Could you check a few things on this model? Use its own coordinates, in mm. A direction names the side the tool comes from. Round coordinates to 2 decimals unless told otherwise and drop trailing zeros. Loops run counter-clockwise (first coordinate to the right, second up) from the corner with the lowest first, then second, coordinate; pieces in that order, holes last. Notation, with made-up numbers: (-31.75, 56.25) - (18.25, 56.25) arc R6 cw to (18.25, 64.25) - close; hole circle Ø6 at (10.5, -8). An arc over 180 degrees is marked (long way). Use one line per item in the form item = value.
```python
from build123d import *

# Parameters (mm, degrees)
SKETCH_1_R      = 3.6
SKETCH_1_R_2    = 2.3
EXTRUDE_1_DEPTH = 5
EXTRUDE_START   = 5
SKETCH_1_8_R    = 3.6
EXTRUDE_2_DEPTH = 20
FILLET_2_R      = 10
FILLET_3_R      = 3


with BuildPart() as part:
    # 草图1 → 凸台-拉伸1 (new body)
    # profile 1 of 5: a face of its own
    with BuildSketch(Plane(origin=(0, 0, 5), x_dir=(1, 0, 0), z_dir=(0, 1, 0))):
        with BuildLine():
            ThreePointArc((13, -81.528896907), (0, -82.5), (-13, -81.528896907))
            Line((-13, -81.528896907), (-13, -94.528896907))
            Line((-13, -94.528896907), (13, -94.528896907))
            Line((13, -94.528896907), (13, -81.528896907))
        make_face()
        with Locations((-8, -89.528896907)):
            Circle(SKETCH_1_R, mode=Mode.SUBTRACT)
        with Locations((8, -89.528896907)):
            Circle(SKETCH_1_R, mode=Mode.SUBTRACT)
    # profile 2 of 5: a face of its own
    with BuildSketch(Plane(origin=(0, 0, 5), x_dir=(1, 0, 0), z_dir=(0, 1, 0))):
        with BuildLine():
            ThreePointArc((-83.157982179, 20), (0, -79.5), (83.157982179, 20))
            Line((83.157982179, 20), (86.204698248, 20))
            ThreePointArc((86.204698248, 20), (0, -82.5), (-86.204698248, 20))
            Line((-86.204698248, 20), (-83.157982179, 20))
        make_face()
    # profile 3 of 5: a face of its own
    with BuildSketch(Plane(origin=(0, 0, 5), x_dir=(1, 0, 0), z_dir=(0, 1, 0))):
        with BuildLine():
            ThreePointArc((13, -81.528896907), (0, -82.5), (-13, -81.528896907))
            Line((-13, -81.528896907), (-13, -94.528896907))
            Line((-13, -94.528896907), (13, -94.528896907))
            Line((13, -94.528896907), (13, -81.528896907))
        make_face()
        with Locations((-8, -89.528896907)):
            Circle(SKETCH_1_R, mode=Mode.SUBTRACT)
        with Locations((8, -89.528896907)):
            Circle(SKETCH_1_R, mode=Mode.SUBTRACT)
    # profile 4 of 5: a face of its own
    with BuildSketch(Plane(origin=(0, 0, 5), x_dir=(1, 0, 0), z_dir=(0, 1, 0))):
        with Locations((-8, -89.528896907)):
            Circle(SKETCH_1_R)
        with Locations(Location((-8, -89.528896907, 0), (0, 0, 270))):
            Circle(SKETCH_1_R_2, mode=Mode.SUBTRACT)
    # profile 5 of 5: a face of its own
    with BuildSketch(Plane(origin=(0, 0, 5), x_dir=(1, 0, 0), z_dir=(0, 1, 0))):
        with Locations((8, -89.528896907)):
            Circle(SKETCH_1_R)
        with Locations(Location((8, -89.528896907, 0), (0, 0, 270))):
            Circle(SKETCH_1_R_2, mode=Mode.SUBTRACT)
    extrude(amount=EXTRUDE_1_DEPTH)

    # 草图1<8> → 凸台-拉伸2 (add)
    # profile 1 of 3: a face of its own
    with BuildSketch(Plane(origin=(0, 0, 5), x_dir=(1, 0, 0), z_dir=(0, 1, 0)).offset(EXTRUDE_START)):
        with BuildLine():
            ThreePointArc((13, -81.528896907), (0, -82.5), (-13, -81.528896907))
            Line((-13, -81.528896907), (-13, -94.528896907))
            Line((-13, -94.528896907), (13, -94.528896907))
            Line((13, -94.528896907), (13, -81.528896907))
        make_face()
        with Locations(Location((-8, -89.528896907, 0), (0, 0, 270))):
            Circle(SKETCH_1_8_R, mode=Mode.SUBTRACT)
        with Locations(Location((8, -89.528896907, 0), (0, 0, 270))):
            Circle(SKETCH_1_8_R, mode=Mode.SUBTRACT)
    # profile 2 of 3: a face of its own
    with BuildSketch(Plane(origin=(0, 0, 5), x_dir=(1, 0, 0), z_dir=(0, 1, 0)).offset(EXTRUDE_START)):
        with BuildLine():
            ThreePointArc((-83.157982179, 20), (0, -79.5), (83.157982179, 20))
            Line((83.157982179, 20), (86.204698248, 20))
            ThreePointArc((86.204698248, 20), (0, -82.5), (-86.204698248, 20))
            Line((-86.204698248, 20), (-83.157982179, 20))
        make_face()
    # profile 3 of 3: a face of its own
    with BuildSketch(Plane(origin=(0, 0, 5), x_dir=(1, 0, 0), z_dir=(0, 1, 0)).offset(EXTRUDE_START)):
        with BuildLine():
            ThreePointArc((13, -81.528896907), (0, -82.5), (-13, -81.528896907))
            Line((-13, -81.528896907), (-13, -94.528896907))
            Line((-13, -94.528896907), (13, -94.528896907))
            Line((13, -94.528896907), (13, -81.528896907))
        make_face()
        with Locations(Location((-8, -89.528896907, 0), (0, 0, 270))):
            Circle(SKETCH_1_8_R, mode=Mode.SUBTRACT)
        with Locations(Location((8, -89.528896907, 0), (0, 0, 270))):
            Circle(SKETCH_1_8_R, mode=Mode.SUBTRACT)
    extrude(amount=EXTRUDE_2_DEPTH)

    # 圆角2
    # the kernel refuses this fillet: 10 mm, written as the material it adds along each edge
    with BuildSketch(Plane(origin=(13, 25, 86.528896907), x_dir=(0, 0, 1), z_dir=(0, -1, 0))) as fillet_2_piece_1:
        with BuildLine():
            CenterArc((8.219454002, -10), FILLET_2_R, 90, 76.355470557)
            ThreePointArc((-1.498325579, -7.641025641), (-0.664124715, -3.837187901), (0, 0))
            Line((0, 0), (8.219454002, 0))
        make_face()
    extrude(amount=25)
    with BuildSketch(Plane(origin=(-13, 25, 86.528896907), x_dir=(-0.9813116821933555, 0, -0.1924250045884026), z_dir=(0, -1, 0))) as fillet_2_piece_2:
        with BuildLine():
            CenterArc((8.231488348, -9.990096279), FILLET_2_R, 92.550190808, 76.355470557)
            Line((-1.581628474, -8.065846233), (0, 0))
            ThreePointArc((0, 0), (3.893271516, -0.086657558), (7.786543032, 0))
        make_face()
    extrude(amount=25)
    # the kernel refuses this fillet: 10 mm, written as the material it takes off along each edge
    with BuildSketch(Plane(origin=(-83.157982179, -17.895247065, -15), x_dir=(-0.13567256273252146, 0, 0.9907537311166635), z_dir=(0, 1, 0))) as fillet_2_2_piece_1:
        with BuildLine():
            CenterArc((7.581654969, -9.991025983), FILLET_2_R, 92.427524139, 43.365844963)
            Line((0.413355777, -3.018545313), (0, 0))
            ThreePointArc((0, 0), (3.579049413, -0.075830444), (7.158098826, 0))
        make_face()
    extrude(amount=60.790494129, mode=Mode.SUBTRACT)
    with BuildSketch(Plane(origin=(83.157982179, -17.895247065, -15), x_dir=(1, 0, 0), z_dir=(0, 1, 0))) as fillet_2_2_piece_2:
        with BuildLine():
            CenterArc((10.92726883, -6.15604485), FILLET_2_R, 142.004143618, 43.365844963)
            ThreePointArc((0.971157612, -7.091913119), (0.560708101, -3.535668449), (0, 0))
            Line((0, 0), (3.046716069, 0))
        make_face()
    extrude(amount=60.790494129, mode=Mode.SUBTRACT)

    # 圆角3
    fillet_3_edges = [part.edges().sort_by_distance(p)[0] for p in [
        (13, 12.5, 99.528896907),
        (-13, 12.5, 99.528896907),
    ]]
    fillet(fillet_3_edges, radius=FILLET_3_R)


solid = part.part
```
1. We'd pull the mould along Z, two halves only. Please class faces 3 (the face through (-7.842, 14.86, 90.932)), 4 (the face through (15.08, 12.68, 88.64)), 5 (the face through (-11, 25, 87)): +Z half, -Z half, draft (parallel to the pull), parting line (faces both ways), or undercut.
Solution:
face_3 = undercut
face_4 = +Z half
face_5 = draft
2. If we section it at D-D, the plane z = 35: Write out the boundary of the cut face in (x, y), plus the area to 3 significant figures.
Solution:
outline = (-80.2, 0) - (-76.91, 0) - (-76.91, 25) - (-80.2, 25) - close; (76.91, 0) - (80.2, 0) - (80.2, 25) - (76.91, 25) - close
area = 164 mm^2
3. For P1, Ø1.5, axis at y = 18, z = 40, coming from the -X side; P2, Ø2, axis at y = 19.5, z = 10.5, coming from the +X side; P3, Ø5, axis at y = 10, z = 62, coming from the +X side, each with a flat end and sliding along its axis, tell me the tip position at first contact or that it passes through.
Solution:
P1 = -78.2
P2 = 86.98
P3 = 64.16
4. If we section it at B-B, the plane x = 8: Write out the boundary of the cut face in (y, z), plus the area to 3 significant figures.
Solution:
outline = (0, 84.12) - (25, 84.12) - (25, 90.93) - (5, 90.93) - (5, 92.23) - (0, 92.23) - close; (0, 96.83) - (5, 96.83) - (5, 98.13) - (25, 98.13) - (25, 99.53) - (0, 99.53) - close
area = 218 mm^2
5. If we section it at A-A, the plane z = 0: Write out the boundary of the cut face in (x, y), plus the area to 3 significant figures.
Solution:
outline = (-87.5, 0) - (-84.5, 0) - (-84.5, 25) - (-87.5, 25) - close; (84.5, 0) - (87.5, 0) - (87.5, 25) - (84.5, 25) - close
area = 150 mm^2
6. On a 3-axis mill with a long thin cutter (end or side, diameter ignored), from which of +Z, -Z, +X, -X, +Y, -Y can I reach the whole of each face in a straight line? I mean faces 1 (the face through (8.158, 14.86, 90.932)), 2 (the face through (8.1, 2.46, 92.23)). Say none if no direction works.
Solution:
face_1 = +Y
face_2 = +Y, -Y
7. If we section it at C-C, the plane y = 22: Write out the boundary of the cut face in (x, z).
Solution:
outline = (-86.2, -15) arc R10 ccw to (-84.13, -7.91) arc R84.5 cw (long way) to (84.13, -7.91) arc R10 ccw to (86.2, -15) arc R87.5 ccw to (20.64, 85.03) arc R10 cw to (13, 94.75) - (13, 96.53) arc R3 ccw to (10, 99.53) - (-10, 99.53) arc R3 ccw to (-13, 96.53) - (-13, 94.75) arc R10 cw to (-20.64, 85.03) arc R87.5 ccw to start; hole circle Ø7.2 at (-8, 94.53); hole circle Ø7.2 at (8, 94.53)
8. Please list where these lines run through material, in increasing order: line 1 along X through (y, z) = (21, 23.5); line 2 along X through (y, z) = (18.75, 36); line 3 along Z through (x, y) = (-10, 3.75).
Solution:
line_1 = -84.29 to -81.17, 81.17 to 84.29
line_2 = -79.75 to -76.45, 76.45 to 79.75
line_3 = 83.91 to 93.39, 95.66 to 99.53
